from build123d import *

# Parameters (mm, degrees)
MIRROREDSKETCH_R = 0.5
PAD_DEPTH        = 0.5
SKETCH_R         = 0.5
PAD001_DEPTH     = 0.5
SKETCH001_R      = 3
PAD002_DEPTH     = 3
FILLET_R         = 0.5
SKETCH002_W      = 0.6
SKETCH002_H      = 2.2
POCKET_DEPTH     = 0.2


with BuildPart() as part:
    # MirroredSketch → Pad (new body)
    with BuildSketch(Plane.XY):
        with BuildLine():
            Line((-2.95804, 0.5), (-3, 0.5))
            ThreePointArc((-4, 1.5), (-3.707107, 0.792893), (-3, 0.5))
            ThreePointArc((-4, 1.5), (-5.5, 3), (-7, 1.5))
            Line((-7, 1.5), (-7, -1.5))
            ThreePointArc((-8, -1.5), (-7.5, -2), (-7, -1.5))
            ThreePointArc((-8, -1.5), (-8.585787, -0.085786), (-10, 0.5))
            ThreePointArc((-10, 0.5), (-12.914214, 0), (-10, -0.5))
            ThreePointArc((-9, -1.5), (-9.292893, -0.792893), (-10, -0.5))
            ThreePointArc((-9, -1.5), (-7.5, -3), (-6, -1.5))
            Line((-6, 1.5), (-6, -1.5))
            ThreePointArc((-5, 1.5), (-5.5, 2), (-6, 1.5))
            ThreePointArc((-5, 1.5), (-4.414214, 0.085786), (-3, -0.5))
            Line((-2.95804, -0.5), (-3, -0.5))
            ThreePointArc((-2.95804, -0.5), (-1.936492, -2.291288), (0, -3))
            Line((0, -3), (0, 3))
            ThreePointArc((0, 3), (-1.936492, 2.291288), (-2.95804, 0.5))
        make_face()
        with Locations((-11.414214, 0)):
            Circle(MIRROREDSKETCH_R, mode=Mode.SUBTRACT)
    extrude(amount=PAD_DEPTH)

    # Sketch → Pad001 (join)
    with BuildSketch(Plane.XY):
        with BuildLine():
            Line((2.95804, 0.5), (3, 0.5))
            ThreePointArc((3, 0.5), (3.707107, 0.792893), (4, 1.5))
            ThreePointArc((7, 1.5), (5.5, 3), (4, 1.5))
            Line((7, 1.5), (7, -1.5))
            ThreePointArc((7, -1.5), (7.5, -2), (8, -1.5))
            ThreePointArc((10, 0.5), (8.585787, -0.085786), (8, -1.5))
            ThreePointArc((10, -0.5), (12.914214, 0), (10, 0.5))
            ThreePointArc((10, -0.5), (9.292893, -0.792893), (9, -1.5))
            ThreePointArc((6, -1.5), (7.5, -3), (9, -1.5))
            Line((6, 1.5), (6, -1.5))
            ThreePointArc((6, 1.5), (5.5, 2), (5, 1.5))
            ThreePointArc((3, -0.5), (4.414214, 0.085786), (5, 1.5))
            Line((2.95804, -0.5), (3, -0.5))
            ThreePointArc((0, -3), (1.936492, -2.291288), (2.95804, -0.5))
            Line((0, -3), (0, 3))
            ThreePointArc((2.95804, 0.5), (1.936492, 2.291288), (0, 3))
        make_face()
        with Locations((11.414214, 0)):
            Circle(SKETCH_R, mode=Mode.SUBTRACT)
    extrude(amount=PAD001_DEPTH)

    # Sketch001 (on Face5 of Pad001) → Pad002 (join)
    with BuildSketch(Plane.XY.offset(0.5)):
        Circle(SKETCH001_R)
    extrude(amount=PAD002_DEPTH)

    # Fillet
    fillet_edges = [part.edges().sort_by_distance(p)[0] for p in [
        (-3, 0, 3.5),
    ]]
    fillet(fillet_edges, radius=FILLET_R)

    # Sketch002 (on Face9 of Fillet) → Pocket (cut)
    with BuildSketch(Plane.XY.offset(3.5)):
        with BuildLine():
            ThreePointArc((-0.6, 1.3), (0, -1.431782), (0.6, 1.3))
            Line((0.6, 1.9), (0.6, 1.3))
            ThreePointArc((-0.6, 1.9), (0, -1.992486), (0.6, 1.9))
            Line((-0.6, 1.9), (-0.6, 1.3))
        make_face()
        with Locations((0, 1.1)):
            Rectangle(SKETCH002_W, SKETCH002_H)
    extrude(amount=-POCKET_DEPTH, mode=Mode.SUBTRACT)


solid = part.part
Here's how the part is built. I have some questions about the finished solid (model axes, mm). A direction names the side the tool comes from. Give positions to 0.01 mm unless a question says otherwise; leave off trailing zeros. Order: outer loops, then holes, each group sorted by start corner. A loop starts at its lowest first (then second) coordinate and runs counter-clockwise, first axis right, second up. Notation, with made-up numbers: (54.5, 73) -> (95.5, 73) arc R19 ccw to (95.5, 102) -> close; hole circle Ø11 at (10, 70.5). An arc over 180 degrees is marked (long way). Use a Markdown table: item, result. Add a question column.
Item 1: Imagine slicing it at B-B on x = -7.5. Please give me the cut outline in (y, z), plus the area to 3 significant figures.
Item 2: Imagine slicing it at D-D on x = 9.25. Please give me the cut outline in (y, z), plus the area to 3 significant figures.
Item 3: Imagine slicing it at A-A on z = 1.95. Please give me the cut outline in (x, y), plus the area to 3 significant figures.
Item 4: If we mould it in two halves opening along X, with no side actions, what happens to faces 4 (the face through (-8.7, -0.7, 0.5)), 5 (the face through (3.699, 0.785, 0.246))? For each: pulls with the +X half, pulls with the -X half, needs draft (parallel to the pull), parting line crosses it, or undercut.
Item 5: Imagine slicing it at C-C on y = 0.25. Give the number of separate pieces and of enclosed holes in the cut face, plus the area to 3 significant figures.
Item 6: I need wall thicknesses on line 1 (X direction, y = -2.25, z = 0.35); line 2 (X direction, y = 0, z = 1.45); line 3 (Z direction, x = 6, y = 1.75). Which ranges of each line are inside material? Lowest first, please.
Item 7: Will these pins go through, and if not, where does the flat tip stop? pin 1 (2 mm diameter, centred on x = 7.5, y = -1, fed in from +Z); pin 2 (2 mm diameter, centred on y = 1.5, z = 3, fed in from -X).
Item 8: For faces 1 (the face through (-4.43, 0.1, 0.25)), 2 (the face through (-12.913, 0.059, 0.246)), 3 (the face through (-8.57, -0.1, 0.25)), which set-ups out of +Z, -Z, +X, -X, +Y, -Y let a thin tool reach every point of the face, with its end or its side?
Data:
| question | item | result |
|---|---|---|
| 1 | outline | (-3, 0) -> (-2, 0) -> (-2, 0.5) -> (-3, 0.5) -> close |
| 1 | area | 0.500 mm² |
| 2 | outline | (-0.84, 0) -> (0.35, 0) -> (0.35, 0.5) -> (-0.84, 0.5) -> close |
| 2 | area | 0.596 mm² |
| 3 | outline | circle Ø6 at (0, 0) |
| 3 | area | 28.3 mm² |
| 4 | face 4 | needs draft |
| 4 | face 5 | undercut |
| 5 | separate pieces | 7 |
| 5 | enclosed holes | 0 |
| 5 | area | 26.0 mm² |
| 6 | line 1 | x = -8.8 to -6.2, -1.98 to 1.98, 6.2 to 8.8 |
| 6 | line 2 | x = -3 to 3 |
| 6 | line 3 | z = 0 to 0.5 |
| 7 | pin 1 | stops at z = 0.5 |
| 7 | pin 2 | stops at x = -2.96 |
| 8 | face 1 | +Z, -Z, -Y |
| 8 | face 2 | +Z, -Z |
| 8 | face 3 | +Z, -Z, +Y |
